For this review, take the finished solid that the model builds, in its own axes (mm). Round coordinates to 2 decimals unless told otherwise and drop trailing zeros. Loops run counter-clockwise (first coordinate to the right, second up) from the corner with the lowest first, then second, coordinate; pieces in that order, holes last. Notation, with made-up numbers: (-16.5, -5.5) -> (-7.5, -5.5) arc R32 ccw to (-7.5, 26.5) -> close; hole circle Ø1 at (50, -38). An arc over 180 degrees is marked (long way). One line per question, with ' | ' between items. Start each with the question number.
1. Wall thickness on line 1 along Y through (x, z) = (7.5, 10); line 2 along Y through (x, z) = (-8.5, 6.5); line 3 along X through (y, z) = (-6.25, 16): over which ranges is each line inside the solid? List them lowest first.
2. Consider section B-B (z = 50). Count the separate pieces of the cut face and the enclosed holes in it, and give its area (3 significant figures).
3. Consider section A-A (y = 0). Write out the cut boundary in (x, z).
4. For pin 1 Ø3 at (x, y) = (-5, 4.5) entering from +Z; pin 2 Ø4 at (x, y) = (7, -1) entering from -Z; pin 3 Ø2 at (y, z) = (-1.5, -13.5) entering from +X; pin 4 Ø1.8 at (y, z) = (-3.5, -6) entering from +X, all flat-tipped, find the tip position at first contact; note any pin that passes through.
```python
from build123d import *

# Parameters (mm, degrees)
SKETCH_1_R      = 1.5
SKETCH_1_R_2    = 2.1
EXTRUDE_1_DEPTH = 60
FILLET_1_R      = 1


with BuildPart() as part:
    # 草图1 → 凸台-拉伸1 (new, symmetric)
    with BuildSketch(Plane.XY):
        Polygon((-10, 10), (-10, 4.8), (-8.34, 3.14), (-8.34, 5.4), (-5.753553391, 5.4), (-3.8, 3.446446609), (-3.8, -3.446446609), (-5.753553391, -5.4), (-8.34, -5.4), (-8.34, -3.14), (-10, -4.8), (-10, -10), (-4.8, -10), (-3.14, -8.34), (-5.4, -8.34), (-5.4, -5.753553391), (-3.446446609, -3.8), (3.446446609, -3.8), (5.4, -5.753553391), (5.4, -8.34), (3.14, -8.34), (4.8, -10), (10, -10), (10, -4.8), (8.34, -3.14), (8.34, -5.4), (5.753553391, -5.4), (3.8, -3.446446609), (3.8, 3.446446609), (5.753553391, 5.4), (8.34, 5.4), (8.34, 3.14), (10, 4.8), (10, 10), (4.8, 10), (3.14, 8.34), (5.4, 8.34), (5.4, 5.753553391), (3.446446609, 3.8), (-3.446446609, 3.8), (-5.4, 5.753553391), (-5.4, 8.34), (-3.14, 8.34), (-4.8, 10), align=None)
        with Locations((-7.5, 7.5)):
            Circle(SKETCH_1_R, mode=Mode.SUBTRACT)
        Circle(SKETCH_1_R_2, mode=Mode.SUBTRACT)
        with Locations(Location((-7.5, -7.5, 0), (0, 0, 180))):
            Circle(SKETCH_1_R, mode=Mode.SUBTRACT)
        with Locations((7.5, -7.5)):
            Circle(SKETCH_1_R, mode=Mode.SUBTRACT)
        with Locations(Location((7.5, 7.5, 0), (0, 0, 180))):
            Circle(SKETCH_1_R, mode=Mode.SUBTRACT)
    extrude(amount=EXTRUDE_1_DEPTH, both=True)

    # 圆角1
    fillet_1_edges = [part.edges().sort_by_distance(p)[0] for p in [
        (10, 10, 0),
        (10, -10, 0),
        (-10, -10, 0),
        (-10, 10, 0),
    ]]
    fillet(fillet_1_edges, radius=FILLET_1_R)


solid = part.part
```
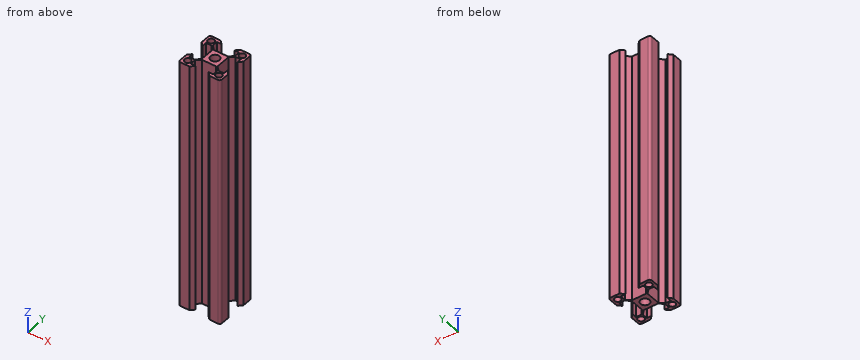
Answer block:
1) line 1: y = -10 to -9, -6 to -5.4, 5.4 to 6, 9 to 10 | line 2: y = -10 to -8.62, -6.38 to -3.3, 3.3 to 6.38, 8.62 to 10 | line 3: x = -10 to -8.33, -6.67 to -5.4, 5.4 to 6.67, 8.33 to 10
2) separate pieces: 1 | enclosed holes: 5 | area: 123 mm2
3) outline: (-3.8, -60) -> (-2.1, -60) -> (-2.1, 60) -> (-3.8, 60) -> close; (2.1, -60) -> (3.8, -60) -> (3.8, 60) -> (2.1, 60) -> close
4) pin 1: stops at z = 60 | pin 2: passes through | pin 3: stops at x = 3.8 | pin 4: stops at x = 9.6
